from build123d import *

# Parameters (mm, degrees)
SKETCH1_W           = 56
SKETCH1_H           = 70
SKETCH1_R           = 1.55
SKETCH1_R_2         = 3.1
BOSS_EXTRUDE1_DEPTH = 2
FILLET1_R           = 3


with BuildPart() as part:
    # Sketch1 → Boss-Extrude1 (new body)
    with BuildSketch(Plane(origin=(0, 0, 0), x_dir=(1, 0, 0), z_dir=(0, 1, 0))):
        Rectangle(SKETCH1_W, SKETCH1_H)
        with Locations((-22.5, -5)):
            Circle(SKETCH1_R, mode=Mode.SUBTRACT)
        with Locations((22.5, -5)):
            Circle(SKETCH1_R, mode=Mode.SUBTRACT)
        with Locations((-4.5, 32)):
            Circle(SKETCH1_R, mode=Mode.SUBTRACT)
        with Locations((4.5, 32)):
            Circle(SKETCH1_R, mode=Mode.SUBTRACT)
        with Locations((-22.5, 10)):
            Circle(SKETCH1_R, mode=Mode.SUBTRACT)
        with Locations((22.5, 10)):
            Circle(SKETCH1_R, mode=Mode.SUBTRACT)
        with Locations((-25, -20)):
            Circle(SKETCH1_R, mode=Mode.SUBTRACT)
        with Locations((25, -20)):
            Circle(SKETCH1_R, mode=Mode.SUBTRACT)
        with Locations((0, -5)):
            Circle(SKETCH1_R_2, mode=Mode.SUBTRACT)
    extrude(amount=BOSS_EXTRUDE1_DEPTH)

    # Fillet1
    fillet1_edges = [part.edges().sort_by_distance(p)[0] for p in [
        (28, 1, 35),
        (-28, 1, 35),
        (-28, 1, -35),
        (28, 1, -35),
    ]]
    fillet(fillet1_edges, radius=FILLET1_R)


solid = part.part
The model under review builds one solid part; all positions refer to its coordinate system, in mm. Round coordinates to 2 decimals unless told otherwise and drop trailing zeros. Order: outer loops, then holes, each group sorted by start corner. A loop starts at its lowest first (then second) coordinate and runs counter-clockwise, first axis right, second up. Notation, with made-up numbers: (-18, -35) - (-8, -35) arc R19 cw to (-8, -9) - close; hole circle Ø9 at (-5.5, -28). An arc over 180 degrees is marked (long way). Use one line per item in the form item = value.
Q1. Clearance check with flat-ended pins moving along their axes: P1, Ø4, axis at x = -22.5, z = 5, coming from the -Y side; P2, Ø1.9, axis at x = -22.5, z = -10, coming from the +Y side. State where each tip first meets the part, or that it passes through.
Response values:
P1 = 0
P2 = through
Q2. Add section B-B on z = 5. Give the boundary of the cut face in (x, y), then the cut area to 3 significant figures.
Response values:
outline = (-28, 0) - (-24.05, 0) - (-24.05, 2) - (-28, 2) - close; (-20.95, 0) - (-3.1, 0) - (-3.1, 2) - (-20.95, 2) - close; (3.1, 0) - (20.95, 0) - (20.95, 2) - (3.1, 2) - close; (24.05, 0) - (28, 0) - (28, 2) - (24.05, 2) - close
area = 87.2 mm^2
Q3. To check wall thickness, follow line 1 (X direction, y = 0.65, z = 20); line 2 (X direction, y = 0.2, z = -10); line 3 (Z direction, x = -22.5, y = 1.05). State the ranges of each line that lie inside material, in increasing order.
Response values:
line_1 = -28 to -26.55, -23.45 to 23.45, 26.55 to 28
line_2 = -28 to -24.05, -20.95 to 20.95, 24.05 to 28
line_3 = -35 to -11.55, -8.45 to 3.45, 6.55 to 35
Q4. Add section A-A on x = -4.5. Give the boundary of the cut face in (y, z).
Response values:
outline = (0, -35) - (2, -35) - (2, -33.55) - (0, -33.55) - close; (0, -30.45) - (2, -30.45) - (2, 35) - (0, 35) - close
Q5. Add section C-C on z = 20. Give the boundary of the cut face in (x, y).
Response values:
outline = (-28, 0) - (-26.55, 0) - (-26.55, 2) - (-28, 2) - close; (-23.45, 0) - (23.45, 0) - (23.45, 2) - (-23.45, 2) - close; (26.55, 0) - (28, 0) - (28, 2) - (26.55, 2) - close
Q6. Mouldability with a two-part tool opening along X and no side actions: class faces 1 (the flat face through (0, 1, 35)), 2 (the cylindrical face through (24.798, 0.986, 18.463)), 3 (the cylindrical face through (-27.14, 1.01, -34.1)) as pulls with the +X half, pulls with the -X half, needs draft (parallel to the pull), parting line crosses it, or undercut.
Response values:
face_1 = needs draft
face_2 = undercut
face_3 = pulls with the -X half
Q7. Add section D-D on y = 0.55. Give the number of separate pieces and of enclosed holes in the cut face, then the cut area to 3 significant figures.
Response values:
separate_pieces = 1
enclosed_holes = 9
area = 3,820 mm^2
